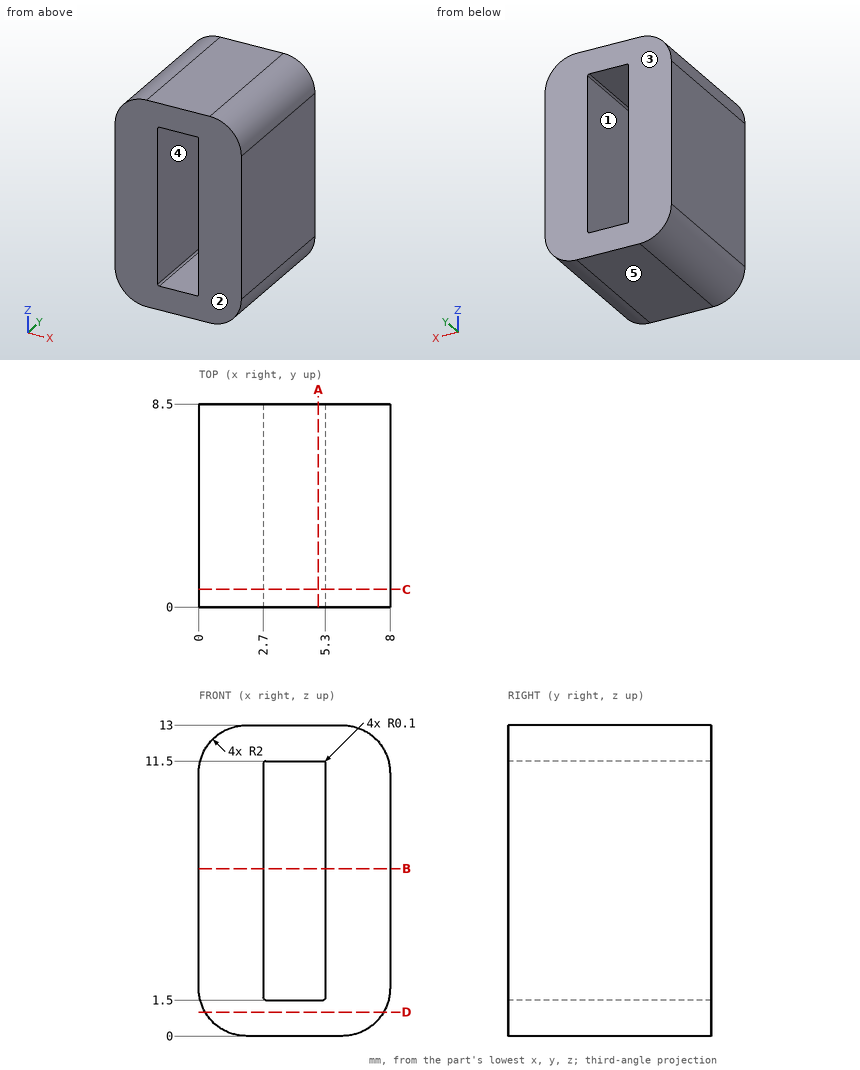
Design review of the part shown in the three views and the two pictorial views. Dimensions are in mm from the part's minimum x, y and z. A direction names the side the tool comes from. Round coordinates to 2 decimals unless told otherwise and drop trailing zeros. Order: outer loops, then holes, each group sorted by start corner. A loop starts at its lowest first (then second) coordinate and runs counter-clockwise, first axis right, second up.
Q1. Machinability: for the marked faces 1 and 2, which of the approach directions +Z, -Z, +X, -X, +Y, -Y give a long, thin tool a straight path to every point of the face, cutting with its end or side? Answer none if there is none.
Findings below:
face 1: +Y, -Y
face 2: +Z, -Z, +X, -X, -Y
Q2. We need section C-C, the plane y = 0.75. Give the boundary of the cut face in (x, z).
Findings below:
outline: (0, 2) arc R2 ccw to (2, 0) - (6, 0) arc R2 ccw to (8, 2) - (8, 11) arc R2 ccw to (6, 13) - (2, 13) arc R2 ccw to (0, 11) - close; hole (2.7, 1.6) arc R0.1 ccw to (2.8, 1.5) - (5.2, 1.5) arc R0.1 ccw to (5.3, 1.6) - (5.3, 11.4) arc R0.1 ccw to (5.2, 11.5) - (2.8, 11.5) arc R0.1 ccw to (2.7, 11.4) - close
Q3. We need section A-A, the plane x = 5. Give the boundary of the cut face in (y, z).
Findings below:
outline: (0, 0) - (8.5, 0) - (8.5, 1.5) - (0, 1.5) - close; (0, 11.5) - (8.5, 11.5) - (8.5, 13) - (0, 13) - close
Q4. Mouldability with a two-part tool opening along Z and no side actions: class the marked faces 3, 4 and 5 as pulls with the +Z half, pulls with the -Z half, needs draft (parallel to the pull), parting line crosses it, or undercut.
Findings below:
face 3: needs draft
face 4: undercut
face 5: pulls with the -Z half
Q5. Wall thickness on line 1 (X direction, y = 4.5, z = 5); line 2 (Z direction, x = 4, y = 2.25); line 3 (Z direction, x = 1.5, y = 1): over which ranges is each line inside the solid? List them lowest first.
Findings below:
line 1: x = 0 to 2.7, 5.3 to 8
line 2: z = 0 to 1.5, 11.5 to 13
line 3: z = 0.06 to 12.94
Q6. We need section D-D, the plane z = 1. Give the boundary of the cut face in (x, y).
Findings below:
outline: (0.27, 0) - (7.73, 0) - (7.73, 8.5) - (0.27, 8.5) - close
Q7. We need section B-B, the plane z = 7. Give the boundary of the cut face in (x, y), plus the area to 3 significant figures.
Findings below:
outline: (0, 0) - (2.7, 0) - (2.7, 8.5) - (0, 8.5) - close; (5.3, 0) - (8, 0) - (8, 8.5) - (5.3, 8.5) - close
area: 45.9 mm2
